Autodesk Inventor part; units mm, degrees
ref_plane "Work Plane2" through (75.376, -18.8821, -44.9646) normal (1, 0, 0) x (0, 1, 0)
ref_plane "Work Plane6" through (0, 25.4, -165.1) normal (0, 0, 1) x (1, 0, 0)
ref_plane "Work Plane10" through (0, 152.4, 0) normal (0, -1, 0) x (1, 0, 0)
sketch "Sketch1" plane through (0, 0, 0) normal (0, 1, 0) x (-1, 0, 0)
  circle A0 centre (0, 0) radius 152.4
  circle A1 centre (0, 0) radius 165.1
  dimension "d0" = 304.8
  dimension "d1" = 330.2
extrude "Extrusion1" add sketch "Sketch1" along normal blind 152.4
sketch "Sketch2" plane through (0, 0, 0) normal (1, 0, 0) x (0, 1, 0)
  circle A0 centre (100.6077, 0) radius 25.4
  point P0 (0, 0)
  dimension "d4" = 50.8
extrude "Extrusion2" add sketch "Sketch2" along normal mid plane 889
sketch "Sketch4" plane through (0, 152.4, 0) normal (0, 1, 0) x (1, 0, 0)
  circle A0 centre (0, 0) radius 152.4
extrude "Extrusion4" cut sketch "Sketch4" against normal through all
sketch "Sketch5" plane through (0, 152.4, 0) normal (0, 1, 0) x (1, 0, 0)
  circle A0 centre (0, 0) radius 165.1
extrude "Extrusion5" add sketch "Sketch5" along normal blind 50.8 draft -50
ref_plane "Work Plane2" through (75.376, -18.8821, -44.9646) normal (1, 0, 0) x (0, 1, 0)
ref_plane "Work Plane5" through (0, 25.4, 165.1) normal (0, 0, 1) x (1, 0, 0)
sketch "Sketch11" plane through (0, 25.4, 165.1) normal (0, 0, 1) x (1, 0, 0)
  circle A0 centre (0, 75.2094) radius 25.4
  line L0 (165.1, -25.4) -> (-165.1, -25.4)
  point P0 (0, -25.4)
  dimension "d31" = 50.8
  dimension "d32" = 100.6094
extrude "Extrusion11" add sketch "Sketch11" along normal blind 280.543
ref_plane "Work Plane6" through (0, 25.4, -165.1) normal (0, 0, 1) x (1, 0, 0)
sketch "Sketch12" plane through (0, 25.4, -165.1) normal (0, 0, 1) x (1, 0, 0)
  circle A0 centre (0, 75.2094) radius 25.4
  line L0 (165.1, -25.4) -> (-165.1, -25.4)
  point P0 (0, -25.4)
  dimension "d36" = 50.8
  dimension "d37" = 100.6094
extrude "Extrusion12" add sketch "Sketch12" against normal blind 280.543
ref_plane "Work Plane10" through (0, 152.4, 0) normal (0, -1, 0) x (1, 0, 0)
ref_plane "Work Plane9" through (0, 63.5, 0) normal (0, -1, 0) x (1, 0, 0)
sketch "Sketch14" plane through (0, 63.5, 0) normal (0, -1, 0) x (1, 0, 0)
  line L0 (-189.7063, -193.5388) -> (215.5754, -193.5388)
  line L1 (215.5754, -193.5388) -> (215.5754, 199.2875)
  line L2 (215.5754, 199.2875) -> (-189.7063, 199.2875)
  line L3 (-189.7063, 199.2875) -> (-189.7063, -193.5388)
  point P0 (0, 0)
extrude "Extrusion14" cut sketch "Sketch14" along normal blind 127
sketch "Sketch15" plane through (0, 152.4, 0) normal (0, -1, 0) x (1, 0, 0)
  line L0 (-561.0288, -551.6284) -> (540.3691, -551.6284)
  line L1 (540.3691, -551.6284) -> (540.3691, 531.8606)
  line L2 (540.3691, 531.8606) -> (-561.0288, 531.8606)
  line L3 (-561.0288, 531.8606) -> (-561.0288, -551.6284)
  point P0 (0, 0)
extrude "Extrusion15" cut sketch "Sketch15" along normal blind 254
ref_plane "Work Plane8" through (0, 0, 0) normal (0, -1, 0) x (1, 0, 0)
properties part number "UpperSailCapTop-ver1-1111-2021"
Check sheet for the modelled part. Datum: model origin and axes. Units: mm. Round coordinates to 2 decimals unless told otherwise and drop trailing zeros. Write each loop counter-clockwise with the first axis right and the second up, starting at its lowest first coordinate (ties: lowest second). Pieces come first, ordered by that corner, then holes. Notation, with made-up numbers: (4, 41) -> (57, 41) arc R6 ccw to (57, 50) -> close; hole circle Ø1 at (8.25, 16). An arc over 180 degrees is marked (long way). Put each result on its own line as item: value.
(1) Sectioned sample at B-B (y = 190). Enter the section's corners in (x, z), plus the area to 3 significant figures.
Values found:
outline: circle Ø240.58 at (0, 0)
area: 45,500 mm^2
(2) Go/stop test with flat-tipped pins: pin 1 Ø3 at (y, z) = (184, 52) entering from -X; pin 2 Ø12 at (y, z) = (172, -40.5) entering from +X; pin 3 Ø6 at (x, y) = (18, 189) entering from +Z. Record where each tip stops, or that it passes through.
Values found:
pin 1: stops at x = -118.41
pin 2: stops at x = 143.46
pin 3: stops at z = 123.78
(3) Sectioned sample at D-D (y = 160.5). Enter the section's corners in (x, z).
Values found:
outline: circle Ø310.89 at (0, 0)
(4) Material ranges on line 1 (Z direction, x = 68.5, y = 186); line 2 (X direction, y = 173, z = -45); line 3 (Y direction, x = -60, z = 89), recorded low to high.
Values found:
line 1: z = -104.63 to 104.63
line 2: x = -133.15 to 133.15
line 3: y = 152.4 to 200.87
(5) Sectioned sample at A-A (x = 0). Enter the section's corners in (y, z), plus the area to 3 significant figures.
Values found:
outline: (152.4, -165.1) -> (203.2, -104.56) -> (203.2, 104.56) -> (152.4, 165.1) -> close
area: 13,700 mm^2
(6) Sectioned sample at C-C (z = 0). Enter the section's corners in (x, y).
Values found:
outline: (-165.1, 152.4) -> (165.1, 152.4) -> (104.56, 203.2) -> (-104.56, 203.2) -> close
